from build123d import *

# Parameters (mm, degrees)
SKETCH1_W           = 80
SKETCH1_H           = 45
BOSS_EXTRUDE1_DEPTH = 25.4
CUT_EXTRUDE5_DEPTH  = 101.6


with BuildPart() as part:
    # Sketch1 → Boss-Extrude1 (new body)
    with BuildSketch(Plane.XY):
        with Locations((-4.545454545, -3.106060606)):
            Rectangle(SKETCH1_W, SKETCH1_H)
    extrude(amount=BOSS_EXTRUDE1_DEPTH)

    # Sketch2 → Cut-Extrude5 (cut)
    with BuildSketch(Plane.ZY.offset(44.545454545)):
        with BuildLine():
            ThreePointArc((21.552264214, 19.393939394), (24.428781954, 9.885974356), (25.4, 0))
            Line((25.4, 0), (25.4, 19.393939394))
            Line((25.4, 19.393939394), (21.552264214, 19.393939394))
        make_face()
        with BuildLine():
            Line((25.4, -25.606060606), (25.4, 0))
            ThreePointArc((25.4, 0), (23.638063736, -13.263042825), (18.474476182, -25.606060606))
            Line((18.474476182, -25.606060606), (25.4, -25.606060606))
        make_face()
    extrude(amount=-CUT_EXTRUDE5_DEPTH, mode=Mode.SUBTRACT)


solid = part.part
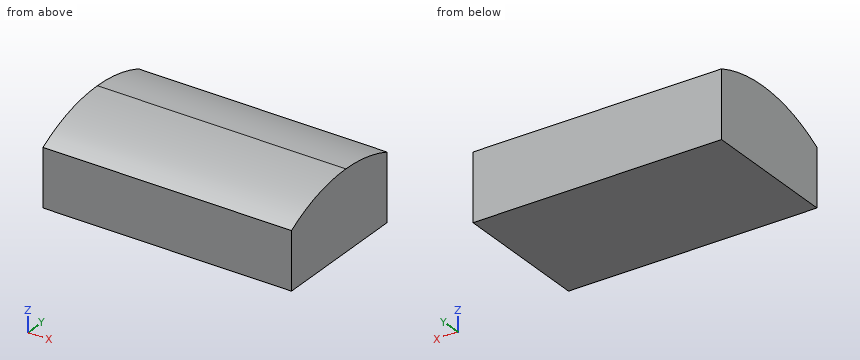
Geometry: final body of the model. Coordinates: model frame, mm. Give positions to 0.01 mm unless a question says otherwise; leave off trailing zeros. Loops run counter-clockwise (first coordinate to the right, second up) from the corner with the lowest first, then second, coordinate; pieces in that order, holes last. Notation, with made-up numbers: M 28.5,65.25 L 52.5,65.25 A22 ccw 52.5,99.25 Z; hole C -10.75,-26.75 d4. An arc over 180 degrees is marked long. Put each result on its own line as item: value.
1) Cut plane A-A, the plane x = -34. Return the cut outline in (y, z), plus the area to 3 significant figures.
Computed values:
outline: M -25.61,0 L 19.39,0 L 19.39,21.55 A50.8 ccw -25.61,18.47 Z
area: 1,060 mm^2
2) Cut plane C-C, the plane y = -10. Return the cut outline in (x, z), plus the area to 3 significant figures.
Computed values:
outline: M -44.55,0 L 35.45,0 L 35.45,24.41 L -44.55,24.41 Z
area: 1,950 mm^2
3) First-contact query: P1, Ø10, axis at x = -35.5, y = -16.5, coming from the +Z side. Flat tip, straight axial feed; report the tip coordinate or a pass-through.
Computed values:
P1: stops at z = 24.08
4) Material intervals for L1, parallel to Z at x = -3.5, y = -17; L2, parallel to Z at x = 27, y = -1.5; L3, parallel to Y at x = -34, z = 19.75, sorted ascending. Write a range as from..to.
Computed values:
L1: z = 0..22.47
L2: z = 0..25.38
L3: y = -23.28..19.39
5) Cut plane B-B, the plane z = 19.25. Return the cut outline in (x, y), plus the area to 3 significant figures.
Computed values:
outline: M -44.55,-24.23 L 35.45,-24.23 L 35.45,19.39 L -44.55,19.39 Z
area: 3,490 mm^2
